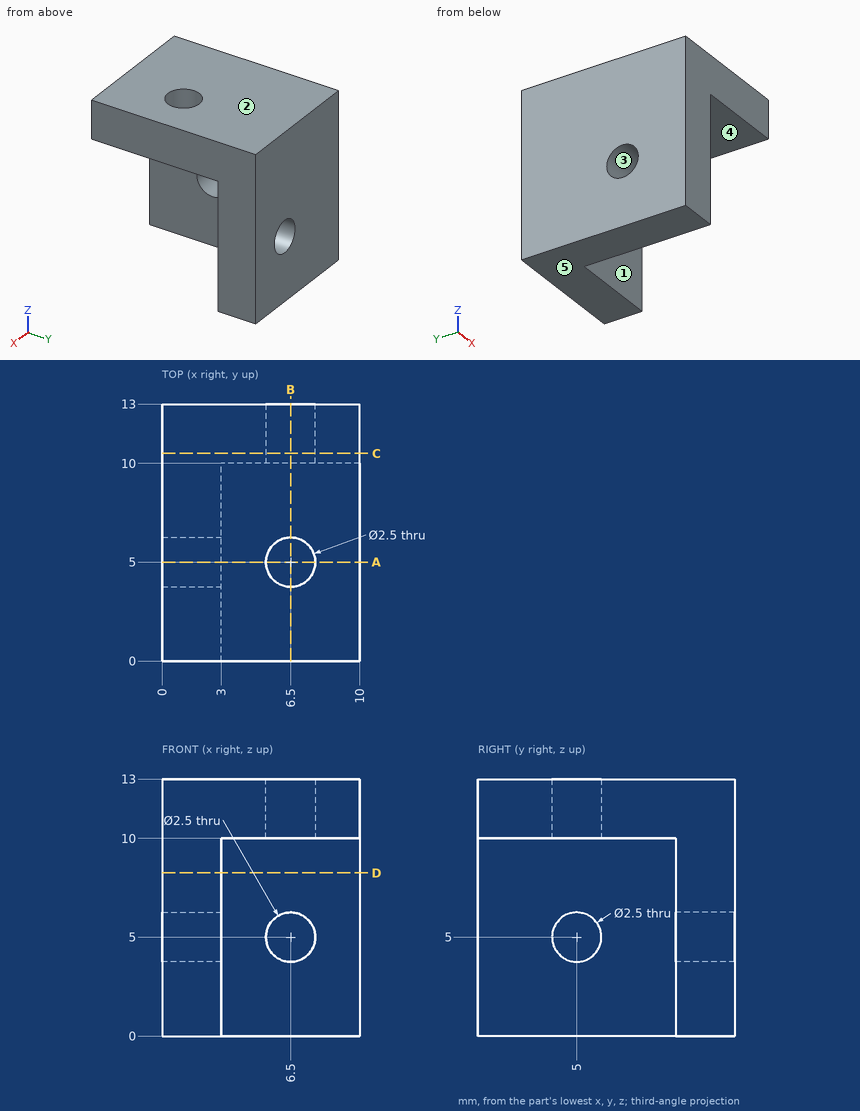
Can you work these out from the drawing? Everything is in mm from the part's minimum corner. A direction names the side the tool comes from. Round coordinates to 2 decimals unless told otherwise and drop trailing zeros. Loops run counter-clockwise (first coordinate to the right, second up) from the corner with the lowest first, then second, coordinate; pieces in that order, holes last. Notation, with made-up numbers: (-31, 50) - (10, 50) arc R23 cw to (10, 89) - close; hole circle Ø10 at (-0.5, 67). An arc over 180 degrees is marked (long way). Answer in a Markdown table with one row per item. Add a question column.
Q1. Which directions (+Z, -Z, +X, -X, +Y, -Y) give clear straight access to the entire face, cutting with the end or side of a thin tool? Please do the marked faces 4 and 5.
Q2. I want a section at B-B on x = 6.5. List the corners of the cut face in (y, z) for me, and give its area (3 significant figures).
Q3. I want a section at C-C on y = 10.5. List the corners of the cut face in (x, z) for me, and give its area (3 significant figures).
Q4. We'd pull the mould along Z, two halves only. Please class the marked faces 1, 2 and 3: pulls with the +Z half, pulls with the -Z half, needs draft (parallel to the pull), parting line crosses it, or undercut.
Q5. I want a section at A-A on y = 5. List the corners of the cut face in (x, z) for me, and give its area (3 significant figures).
Q6. For pin 1 Ø2 at (y, z) = (3, 1.5) entering from +X; pin 2 Ø3.5 at (x, y) = (6, 3.5) entering from -Z; pin 3 Ø1 at (x, z) = (6.5, 3) entering from -Y; pin 4 Ø2 at (x, z) = (6.5, 5) entering from +Y, each with a flat end and sliding along its axis, tell me the tip position at first contact or that it passes through.
Q7. I need wall thicknesses on L1, parallel to Y at x = 0.9, z = 5; L2, parallel to X at y = 5, z = 11.1; L3, parallel to X at y = 6.75, z = 1.25. Which ranges of each line are inside material? Lowest first, please.
Q8. I want a section at D-D on z = 8.25. List the corners of the cut face in (x, y) for me.
A:
| question | item | result |
|---|---|---|
| 1 | face 4 | -Z, +X, -Y |
| 1 | face 5 | -Z, +X, -X, +Y, -Y |
| 2 | outline | (0, 10) - (3.75, 10) - (3.75, 13) - (0, 13) - close; (6.25, 10) - (10, 10) - (10, 6.25) - (13, 6.25) - (13, 13) - (6.25, 13) - close; (10, 0) - (13, 0) - (13, 3.75) - (10, 3.75) - close |
| 2 | area | 54.0 mm^2 |
| 3 | outline | (0, 0) - (10, 0) - (10, 13) - (0, 13) - close; hole circle Ø2.5 at (6.5, 5) |
| 3 | area | 125 mm^2 |
| 4 | face 1 | needs draft |
| 4 | face 2 | pulls with the +Z half |
| 4 | face 3 | undercut |
| 5 | outline | (0, 0) - (3, 0) - (3, 3.75) - (0, 3.75) - close; (0, 6.25) - (3, 6.25) - (3, 10) - (5.25, 10) - (5.25, 13) - (0, 13) - close; (7.75, 10) - (10, 10) - (10, 13) - (7.75, 13) - close |
| 5 | area | 45.0 mm^2 |
| 6 | pin 1 | x = 3 |
| 6 | pin 2 | z = 10 |
| 6 | pin 3 | y = 10 |
| 6 | pin 4 | through |
| 7 | L1 | 0 to 3.75, 6.25 to 13 |
| 7 | L2 | 0 to 5.25, 7.75 to 10 |
| 7 | L3 | 0 to 3 |
| 8 | outline | (0, 0) - (3, 0) - (3, 10) - (10, 10) - (10, 13) - (0, 13) - close |
